Geometry check sheet. Reference: the model listing, model coordinates, mm. A direction names the side the tool comes from. Round coordinates to 2 decimals unless told otherwise and drop trailing zeros. Order: outer loops, then holes, each group sorted by start corner. A loop starts at its lowest first (then second) coordinate and runs counter-clockwise, first axis right, second up. Notation, with made-up numbers: (85, 7.25) - (102, 7.25) arc R7 ccw to (102, 15.25) - close; hole circle Ø4 at (66, 61). An arc over 180 degrees is marked (long way). Use a Markdown table: item, result. Add a question column.
(1) Access from +Z, -Z, +X, -X, +Y, -Y to the whole of each face (thin tool, end or side, straight path). Record for faces 3 (the face through (-8, -2, -12)), 4 (the face through (10.146, 3.456, -1.39)), 5 (the face through (0, -4, -25)).
(2) Mould release check, pull along Z, two halves, no side actions. Record for faces 1 (the face through (13.003, 8.014, -13.068)), 2 (the face through (12, 3, -12)): released by +Z, released by -Z, zero draft, split by the parting line, or undercut.
(3) Section check A-A on y = -0.75. Record the boundary of the cut face in (x, z).
(4) Thickness scan on line 1 along Y through (x, z) = (-4.75, -20); line 2 along X through (y, z) = (3.9, -15.5) (3 decimals); line 3 along Z through (x, y) = (12.5, 3.75). Record the ranges inside material, lowest first. Write a range as [from, to].
(5) Section check B-B on z = -4. Give the number of separate pieces and of enclosed holes in the cut face, then the cut area to 3 significant figures.
(6) Gauge pin test, flat ends, axial feed: P1, Ø3, axis at x = 11.625, z = -4, coming from the -Y side; P2, Ø2.5, axis at x = -10.5, z = -11.5, coming from the -Y side; P3, Ø7, axis at y = -3.5, z = -12.5, coming from the -X side; P4, Ø1.5, axis at y = 6, z = -13.5, coming from the +X side (3 decimals). Record the tip position at first contact, or that the pin passes through.
(7) Section check C-C on x = 0. Record the boundary of the cut face in (y, z), then the cut area to 3 significant figures.
(8) Section check D-D on y = 4.5. Record the boundary of the cut face in (x, z) (3 decimals).
```python
from build123d import *

# Parameters (mm, degrees)
EXTRUDE_1_DEPTH          = 2
EXTRUDE_2_DEPTH          = 26
SKETCH_3_W               = 12
SKETCH_3_H               = 1
EXTRUDE_3_DEPTH          = 1.6
CUT_EXTRUDE_1_DEPTH      = 2
CUT_EXTRUDE_2_DEPTH      = 11
CUT_EXTRUDE_2_DEPTH_BACK = 0.5
CUT_EXTRUDE_3_DEPTH      = 11
CUT_EXTRUDE_3_DEPTH_BACK = 1
SKETCH_7_R               = 1.35
SKETCH_7_R_2             = 1.6
CUT_EXTRUDE_4_DEPTH      = 1
CUT_EXTRUDE_4_DEPTH_BACK = 6


with BuildPart() as part:
    # 草图1 → 凸台-拉伸1 (new body)
    with BuildSketch(Plane.XY):
        with BuildLine():
            ThreePointArc((8, 2), (8.292893219, 2.707106781), (9, 3))
            Line((9, 3), (15, 3))
            ThreePointArc((15, 3), (15.707106781, 3.292893219), (16, 4))
            Line((16, 4), (16, 8))
            ThreePointArc((16, 8), (15.707106781, 8.707106781), (15, 9))
            Line((15, 9), (-12.875, 9))
            ThreePointArc((-12.875, 9), (-13.582106781, 8.707106781), (-13.875, 8))
            Line((-13.875, 8), (-13.875, 4))
            ThreePointArc((-13.875, 4), (-13.582106781, 3.292893219), (-12.875, 3))
            Line((-12.875, 3), (-8, 3))
            Line((-8, 3), (-8, -6))
            ThreePointArc((-8, -6), (-7.707106781, -6.707106781), (-7, -7))
            Line((-7, -7), (7, -7))
            ThreePointArc((7, -7), (7.707106781, -6.707106781), (8, -6))
            Line((8, -6), (8, 2))
        make_face()
        with BuildLine():
            Line((4, -5), (-4, -5))
            Line((-4, -5), (-4, 0))
            ThreePointArc((-4, 0), (0, 4), (4, 0))
            Line((4, 0), (4, -5))
        make_face(mode=Mode.SUBTRACT)
    extrude(amount=EXTRUDE_1_DEPTH)

    # 草图2 → 凸台-拉伸2 (add)
    with BuildSketch(Plane(origin=(0, 0, 0), x_dir=(-1, 0, 0), z_dir=(0, 0, -1))):
        with BuildLine():
            Line((6, -4), (6, -5))
            Line((6, -5), (5, -5))
            Line((5, -5), (-5, -5))
            Line((-5, -5), (-6, -5))
            Line((-6, -5), (-6, -4))
            Line((-6, -4), (-6, 4))
            Line((-6, 4), (-6, 5))
            Line((-6, 5), (-16, 5))
            Line((-16, 5), (-16, 4))
            ThreePointArc((-16, 4), (-15.707106781, 3.292893219), (-15, 3))
            Line((-15, 3), (-9, 3))
            ThreePointArc((-9, 3), (-8.292893219, 2.707106781), (-8, 2))
            Line((-8, 2), (-8, -6))
            ThreePointArc((-8, -6), (-7.707106781, -6.707106781), (-7, -7))
            Line((-7, -7), (7, -7))
            ThreePointArc((7, -7), (7.707106781, -6.707106781), (8, -6))
            Line((8, -6), (8, 3))
            Line((8, 3), (12.875, 3))
            ThreePointArc((12.875, 3), (13.582106781, 3.292893219), (13.875, 4))
            Line((13.875, 4), (13.875, 8))
            ThreePointArc((13.875, 8), (13.582106781, 8.707106781), (12.875, 9))
            Line((12.875, 9), (-15, 9))
            ThreePointArc((-15, 9), (-15.707106781, 8.707106781), (-16, 8))
            Line((-16, 8), (-16, 7))
            Line((-16, 7), (11.875, 7))
            Line((11.875, 7), (11.875, 5))
            Line((11.875, 5), (6, 5))
            Line((6, 5), (6, 4))
            Line((6, 4), (6, -4))
        make_face()
    extrude(amount=EXTRUDE_2_DEPTH)

    # 草图3 → 凸台-拉伸3 (add)
    with BuildSketch(Plane(origin=(0, 0, -26), x_dir=(-1, 0, 0), z_dir=(0, 0, -1))):
        with Locations((0, -4.5)):
            Rectangle(SKETCH_3_W, SKETCH_3_H)
    extrude(amount=-EXTRUDE_3_DEPTH)

    # 草图4 → 切除-拉伸1 (cut)
    with BuildSketch(Plane(origin=(0, 9, 0), x_dir=(1, 0, 0), z_dir=(0, 1, 0))):
        Polygon((11.625, 12.272649731), (14.41996732, 13.886324865), (14.41996732, 17.113675135), (11.625, 18.727350269), (8.83003268, 17.113675135), (8.83003268, 13.886324865), align=None)
    extrude(amount=-CUT_EXTRUDE_1_DEPTH, mode=Mode.SUBTRACT)

    # 草图5 → 切除-拉伸2 (cut, two sides)
    with BuildSketch(Plane.XZ.offset(-3)) as cut_extrude_2_sk:
        Polygon((11.625, -18.675426481), (14.375, -17.08771324), (14.375, -13.91228676), (11.625, -12.324573519), (8.875, -13.91228676), (8.875, -17.08771324), align=None)
    extrude(amount=CUT_EXTRUDE_2_DEPTH, mode=Mode.SUBTRACT)
    extrude(cut_extrude_2_sk.sketch, amount=-CUT_EXTRUDE_2_DEPTH_BACK, mode=Mode.SUBTRACT)

    # 草图6 → 切除-拉伸3 (cut, two sides)
    with BuildSketch(Plane.XZ.offset(-3)) as cut_extrude_3_sk:
        Polygon((8.625, -5.732050808), (11.625, -7.464101615), (14.625, -5.732050808), (14.625, -2.267949192), (11.625, -0.535898385), (8.625, -2.267949192), align=None)
    extrude(amount=CUT_EXTRUDE_3_DEPTH, mode=Mode.SUBTRACT)
    extrude(cut_extrude_3_sk.sketch, amount=-CUT_EXTRUDE_3_DEPTH_BACK, mode=Mode.SUBTRACT)

    # 草图7 → 切除-拉伸4 (cut, two sides)
    with BuildSketch(Plane.XZ.offset(-4)) as cut_extrude_4_sk:
        with Locations((11.625, -15.5)):
            Circle(SKETCH_7_R)
        with Locations((11.625, -4)):
            Circle(SKETCH_7_R_2)
    extrude(amount=CUT_EXTRUDE_4_DEPTH, mode=Mode.SUBTRACT)
    extrude(cut_extrude_4_sk.sketch, amount=-CUT_EXTRUDE_4_DEPTH_BACK, mode=Mode.SUBTRACT)


solid = part.part
```
Check sheet entries:
| question | item | result |
|---|---|---|
| 1 | face 3 | +Z, -Z, -X, -Y |
| 1 | face 4 | -Y |
| 1 | face 5 | -Z |
| 2 | face 1 | undercut |
| 2 | face 2 | zero draft |
| 3 | outline | (-8, -26) - (-6, -26) - (-6, 0) - (-4, 0) - (-4, 2) - (-8, 2) - close; (4, 0) - (6, 0) - (6, -26) - (8, -26) - (8, 2) - (4, 2) - close |
| 4 | line 1 | y = [-7, -5], [7, 9] |
| 4 | line 2 | x = [-13.87, -6], [6, 10.275], [12.975, 15.995] |
| 4 | line 3 | z = [-26, -16.53], [-14.47, -6.96], [-1.04, 2] |
| 5 | separate pieces | 3 |
| 5 | enclosed holes | 0 |
| 5 | area | 147 mm2 |
| 6 | P1 | passes through |
| 6 | P2 | stops at y = 3 |
| 6 | P3 | stops at x = -8 |
| 6 | P4 | stops at x = -11.875 |
| 7 | outline | (-7, -26) - (-4, -26) - (-4, -24.4) - (-5, -24.4) - (-5, 2) - (-7, 2) - close; (4, 0) - (7, 0) - (7, -26) - (9, -26) - (9, 2) - (4, 2) - close |
| 7 | area | 120 mm2 |
| 8 | outline | (-13.875, -26) - (-6, -26) - (-6, 0) - (6, 0) - (6, -26) - (16, -26) - (16, 2) - (-13.875, 2) - close; hole circle Ø3.2 at (11.625, -4); hole circle Ø2.7 at (11.625, -15.5) |
